Source: CAD feature listing. Evaluate the final solid. Frame: model axes, mm. A direction names the side the tool comes from. Give positions to 0.01 mm unless a question says otherwise; leave off trailing zeros. Order: outer loops, then holes, each group sorted by start corner. A loop starts at its lowest first (then second) coordinate and runs counter-clockwise, first axis right, second up.
1) First-contact query: P1, Ø12, axis at x = 19, y = -3.5, coming from the -Z side; P2, Ø3, axis at x = 17.5, z = -8.5, coming from the -Y side; P3, Ø0.7, axis at x = 17, y = -3, coming from the +Z side. Flat tips, straight axial feed; report the tip coordinate or a pass-through.
2) Section D-D, the plane x = 17.5. Give the number of separate pieces and of enclosed holes in the cut face, plus the area to 3 significant figures.
3) Draft query along Z for faces 1 (the face through (17, -25.5, -29)), 2 (the face through (17, -22, -38)), 3 (the face through (19.87, -2.817, -9.394)). Return one class per face: released by +Z, released by -Z, zero draft, split by the parting line, or undercut.
4) Material intervals for line 1 (Z direction, x = 16, y = -24.5); line 2 (Z direction, x = 3, y = -21); line 3 (Z direction, x = 13.5, y = -2.5), sorted ascending.
5) Section A-A, the plane x = 6. Return loops of the section in (y, z), plus the area to 3 significant figures.
6) Access query for faces 4 (the face through (18.9, -1.6, -6.7)), 5 (the face through (17, -4, 0)), 6 (the face through (18, -20, -35.55)), 7 (the face through (17, -23, -34.25)). Directions: +Z, -Z, +X, -X, +Y, -Y. A direction counts if a zero-diameter tool reaches every point of the face in a straight line with its end or side. Return the directions, or none.
7) Section C-C, the plane z = -1.5. Return loops of the section in (x, y) (3 decimals), plus the area to 3 significant figures.
8) Section B-B, the plane y = -7.25. Return loops of the section in (x, z).
```python
from build123d import *

# Parameters (mm, degrees)
SALIENTE_EXTRUIR1_DEPTH = 35
CORTAR_EXTRUIR1_DEPTH   = 8.5
CROQUIS3_R              = 1.75
CORTAR_EXTRUIR2_DEPTH   = 26.5
CORTAR_EXTRUIR3_DEPTH   = 2.4
CORTAR_EXTRUIR4_DEPTH   = 3.5
CROQUIS8_R              = 1.575
CORTAR_EXTRUIR6_DEPTH   = 5


with BuildPart() as part:
    # Croquis1 → Saliente-Extruir1 (new body)
    with BuildSketch(Plane(origin=(0, 0, 0), x_dir=(0, 0, -1), z_dir=(1, 0, 0))):
        Polygon((-38, -18), (-27, -18), (-27, 0), (27, 0), (27, -18), (38, -18), (38, -25.5), (23, -25.5), (23, -4), (-23, -4), (-23, -25.5), (-38, -25.5), align=None)
    extrude(amount=SALIENTE_EXTRUIR1_DEPTH)

    # Croquis2 → Cortar-Extruir1 (cut, through all)
    with BuildSketch(Plane(origin=(0, -18, 0), x_dir=(1, 0, 0), z_dir=(0, 1, 0))):
        with BuildLine():
            Line((4.5, 34.25), (30.5, 34.25))
            ThreePointArc((30.5, 34.25), (32.75, 32), (30.5, 29.75))
            Line((30.5, 29.75), (4.5, 29.75))
            ThreePointArc((4.5, 29.75), (2.25, 32), (4.5, 34.25))
        make_face()
        with BuildLine():
            Line((4.5, -29.75), (30.5, -29.75))
            ThreePointArc((30.5, -29.75), (32.75, -32), (30.5, -34.25))
            Line((30.5, -34.25), (4.5, -34.25))
            ThreePointArc((4.5, -34.25), (2.25, -32), (4.5, -29.75))
        make_face()
    extrude(amount=-CORTAR_EXTRUIR1_DEPTH, mode=Mode.SUBTRACT)

    # Croquis3 → Cortar-Extruir2 (cut, through all)
    with BuildSketch(Plane(origin=(0, 0, 0), x_dir=(1, 0, 0), z_dir=(0, 1, 0))):
        with Locations((17.5, 18)):
            Circle(CROQUIS3_R)
        with Locations((17.5, 8)):
            Circle(CROQUIS3_R)
    extrude(amount=-CORTAR_EXTRUIR2_DEPTH, mode=Mode.SUBTRACT)

    # Croquis4 → Cortar-Extruir3 (cut)
    with BuildSketch(Plane.XZ.offset(4)):
        Polygon((20.675426481, -8), (19.08771324, -5.25), (15.91228676, -5.25), (14.324573519, -8), (15.91228676, -10.75), (19.08771324, -10.75), align=None)
        Polygon((20.675426481, -18), (19.08771324, -15.25), (15.91228676, -15.25), (14.324573519, -18), (15.91228676, -20.75), (19.08771324, -20.75), align=None)
    extrude(amount=-CORTAR_EXTRUIR3_DEPTH, mode=Mode.SUBTRACT)

    # Croquis5 → Cortar-Extruir4 (cut)
    with BuildSketch(Plane.XZ.offset(18)):
        Polygon((0.400813089, -32), (2.450406544, -28.45), (32.549593456, -28.45), (34.599186911, -32), (32.549593456, -35.55), (2.450406544, -35.55), align=None)
        Polygon((0.400813089, 32), (2.450406544, 28.45), (32.549593456, 28.45), (34.599186911, 32), (32.549593456, 35.55), (2.450406544, 35.55), align=None)
    extrude(amount=CORTAR_EXTRUIR4_DEPTH, mode=Mode.SUBTRACT)

    # Croquis8 → Cortar-Extruir6 (cut, through all)
    with BuildSketch(Plane.XZ.offset(4)):
        with Locations((25, 9)):
            Circle(CROQUIS8_R)
        with Locations((13.615580823, 20.384419177)):
            Circle(CROQUIS8_R)
        with Locations((13.615580823, 16.884419177)):
            Circle(CROQUIS8_R)
        with Locations((25, 5.5)):
            Circle(CROQUIS8_R)
        with Locations((13.615580823, 13.384419177)):
            Circle(CROQUIS8_R)
        with Locations((25, 2)):
            Circle(CROQUIS8_R)
        with Locations((13.615580823, 9.884419177)):
            Circle(CROQUIS8_R)
        with Locations((25, -1.5)):
            Circle(CROQUIS8_R)
        with Locations((13.615580823, 6.384419177)):
            Circle(CROQUIS8_R)
        with Locations((25, -5)):
            Circle(CROQUIS8_R)
    extrude(amount=-CORTAR_EXTRUIR6_DEPTH, mode=Mode.SUBTRACT)


solid = part.part
```
From the geometry:
1. P1: stops at z = -27
1. P2: stops at y = -1.6
1. P3: stops at z = 27
2. separate pieces: 5
2. enclosed holes: 0
2. area: 430 mm2
3. face 1: zero draft
3. face 2: released by -Z
3. face 3: undercut
4. line 1: z = -38 to -34.25, -29.75 to -23, 23 to 29.75, 34.25 to 38
4. line 2: z = -38 to -35.55, -28.45 to -23, 23 to 28.45, 35.55 to 38
4. line 3: z = -27 to 4.81, 7.96 to 8.31, 11.46 to 11.81, 14.96 to 15.31, 18.46 to 18.81, 21.96 to 27
5. outline: (-25.5, -38) - (-18, -38) - (-18, -35.55) - (-21.5, -35.55) - (-21.5, -34.25) - (-25.5, -34.25) - close; (-25.5, -29.75) - (-21.5, -29.75) - (-21.5, -28.45) - (-18, -28.45) - (-18, -27) - (0, -27) - (0, 27) - (-18, 27) - (-18, 28.45) - (-21.5, 28.45) - (-21.5, 29.75) - (-25.5, 29.75) - (-25.5, 23) - (-4, 23) - (-4, -23) - (-25.5, -23) - close; (-25.5, 34.25) - (-21.5, 34.25) - (-21.5, 35.55) - (-18, 35.55) - (-18, 38) - (-25.5, 38) - close
5. area: 467 mm2
6. face 4: -Y
6. face 5: +X, -X, -Y
6. face 6: +Y
6. face 7: +Y, -Y
7. outline: (0, -4) - (23.425, -4) - (23.425, 0) - (0, 0) - close; (26.575, -4) - (35, -4) - (35, 0) - (26.575, 0) - close
7. area: 127 mm2
8. outline: (0, -27) - (35, -27) - (35, -23) - (0, -23) - close; (0, 23) - (35, 23) - (35, 27) - (0, 27) - close
